Input: dimensioned drawing with shaded views. Units: mm. Origin: part minimum x, y, z. Coordinates: 2 decimals unless noted, no trailing zeros. Use CSV: the item, a comma, the result in double quotes. Start each with the question number.
1. Section query A-A on y = 76.3. State how many separate pieces and enclosed holes the cut face has, and give its area (3 significant figures).
2. First-contact query: P1, Ø3, axis at x = 12.2, y = 38, coming from the +Z side. Flat tip, straight axial feed; report the tip coordinate or a pass-through.
3. Material intervals for line 1 (Y direction, x = 70, z = 2.5); line 2 (Y direction, x = 64, z = 7.75); line 3 (X direction, y = 76.3, z = 5.5), sorted ascending.
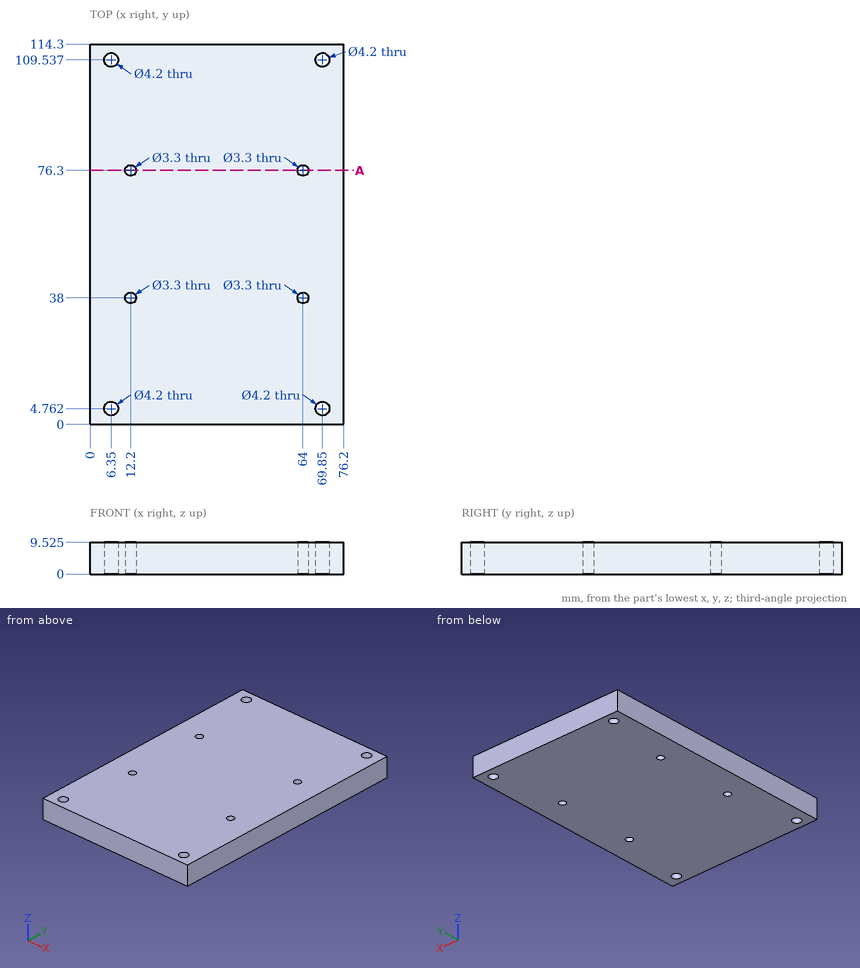
Results list:
1,separate pieces,"3"
1,enclosed holes,"0"
1,area,"663 mm²"
2,P1,"passes through"
3,line 1,"y = 0 to 2.67, 6.86 to 107.44, 111.63 to 114.3"
3,line 2,"y = 0 to 36.35, 39.65 to 74.65, 77.95 to 114.3"
3,line 3,"x = 0 to 10.55, 13.85 to 62.35, 65.65 to 76.2"
